```python
from build123d import *

# Parameters (mm, degrees)
F0_W = 72.6
F0_H = 3.9
F2_R = 0.8
F3_R = 0.4


with BuildPart() as f1:
    # F0 (on Top) → F1 (revolve)
    with BuildSketch(Plane.XY):
        Polygon((-12.7115285009, 12.0947610609), (-16.1115285009, 10.8947610609), (-12.7115285009, 10.8947610609), align=None)
        Polygon((-7.7115285009, 10.8947610609), (-7.7115285009, 13.1447610609), (-12.7115285009, 13.1447610609), (-12.7115285009, 12.0947610609), (-12.7115285009, 10.8947610609), align=None)
        Polygon((-3.7115285009, 10.8947610609), (-3.7115285009, 14.7947610609), (-7.7115285009, 13.1447610609), (-7.7115285009, 10.8947610609), align=None)
        with Locations((32.5884714991, 12.8447610609)):
            Rectangle(F0_W, F0_H)
    revolve(axis=Axis((26.3884714991, 10.8947610609, 0), (-1, 0, 0)))

    # F2
    f2_edges = [f1.edges().sort_by_distance(p)[0] for p in [
        (68.888471, 6.994761, 0),
    ]]
    fillet(f2_edges, radius=F2_R)

    # F3
    f3_edges = [f1.edges().sort_by_distance(p)[0] for p in [
        (-12.711529, 8.644761, 0),
    ]]
    fillet(f3_edges, radius=F3_R)


solid = f1.part
```
Build history of the part. All positions in model axes, mm. A direction names the side the tool comes from. Give positions to 0.01 mm unless a question says otherwise; leave off trailing zeros. Loops run counter-clockwise (first coordinate to the right, second up) from the corner with the lowest first, then second, coordinate; pieces in that order, holes last.
Item 1: Slice it at A-A, the plane x = 49. List the corners of the cut face in (y, z).
Answers follow:
outline: circle Ø7.8 at (10.89, 0)
Item 2: Which spindle directions (+Z, -Z, +X, -X, +Y, -Y) get a long thin tool onto all of the face, cutting with end or side? Do faces 1 (the face through (-10.044, 8.647, -0.099)), 2 (the face through (68.888, 11, 0)). Say none if no direction does.
Answers follow:
face 1: -X
face 2: +Z, -Z, +X, +Y, -Y
Item 3: Flat gauge pins, fed straight in: pin 1 (1.5 mm diameter, centred on x = -4.5, z = 2, fed in from +Y); pin 2 (1 mm diameter, centred on x = 1, y = 11.5, fed in from +Z); pin 3 (4 mm diameter, centred on y = 12.5, z = 3, fed in from -X). Where does each tip first touch, or does it go through?
Answers follow:
pin 1: stops at y = 14.39
pin 2: stops at z = 3.9
pin 3: stops at x = -12.71
Item 4: Drill centre lines: line 1 (Z direction, x = 51.5, y = 11.25); line 2 (Y direction, x = 62, z = 0.5); line 3 (X direction, y = 10.25, z = -1). Where is each one in solid material? Low to high.
Answers follow:
line 1: z = -3.88 to 3.88
line 2: y = 7.03 to 14.76
line 3: x = -12.74 to 68.89
Item 5: Slice it at B-B, the plane x = -11. List the corners of the cut face in (y, z), and give its area (3 significant figures).
Answers follow:
outline: circle Ø4.5 at (10.89, 0)
area: 15.9 mm2
